Here's how the part is built. I have some questions about the finished solid (model axes, mm). Face numbers are marked on the shaded views. A direction names the side the tool comes from. Coordinates: 2 decimals unless noted, no trailing zeros. Write each loop counter-clockwise with the first axis right and the second up, starting at its lowest first coordinate (ties: lowest second). Pieces come first, ordered by that corner, then holes. Notation, with made-up numbers: (42.25, 3.25) -> (70.25, 3.25) arc R6 ccw to (70.25, 11.25) -> close; hole circle Ø10 at (-21, 64). An arc over 180 degrees is marked (long way). Use CSV: the item, a comma, the result in double quotes. Start each with the question number.
```python
from build123d import *

# Parameters (mm, degrees)
F0_R     = 11.125
F1_DEPTH = 7
F2_DEPTH = 7
F3_DEPTH = 7


with BuildPart() as f1:
    # F0 (on Top) → F1 (new body)
    with BuildSketch(Plane.XY):
        with BuildLine():
            Line((14.352928, 23.6), (0.942339, 49.019534))
            Line((0.942339, 49.019534), (-6.80188, 35.797903))
            Line((-6.80188, 35.797903), (-14.258011, 23.764401))
            Line((-14.258011, 23.764401), (-9.599727, 15.550613))
            ThreePointArc((-9.599727, 15.550613), (-8.984191, 12.491637), (-10.302184, 9.663366))
            ThreePointArc((-10.302184, 9.663366), (-12.214839, 7.093189), (-13.499103, 4.158105))
            ThreePointArc((-13.499103, 4.158105), (-15.307655, 1.607595), (-18.277547, 0.63))
            Line((-18.277547, 0.63), (-27.614663, 0.63))
            Line((-27.614663, 0.63), (-42.923331, -23.693677))
            Line((-42.923331, -23.693677), (-27.600953, -23.789553))
            Line((-27.600953, -23.789553), (-13.45157, -24.23))
            Line((-13.45157, -24.23), (-8.667362, -16.088915))
            ThreePointArc((-8.667362, -16.088915), (-6.325979, -14.026356), (-3.217628, -13.753636))
            ThreePointArc((-3.217628, -13.753636), (-0.035463, -14.124955), (3.148527, -13.769619))
            ThreePointArc((3.148527, -13.769619), (6.261609, -14.060615), (8.593178, -16.14382))
            Line((8.593178, -16.14382), (13.261736, -24.23))
            Line((13.261736, -24.23), (41.980992, -25.325857))
            Line((41.980992, -25.325857), (27.70958, 0.465599))
            Line((27.70958, 0.465599), (18.26709, 0.538301))
            ThreePointArc((18.26709, 0.538301), (15.31017, 1.534719), (13.519812, 4.09027))
            ThreePointArc((13.519812, 4.09027), (12.250302, 7.031766), (10.350576, 9.611514))
            ThreePointArc((10.350576, 9.611514), (9.046046, 12.45302), (9.68437, 15.51382))
            Line((9.68437, 15.51382), (14.352928, 23.6))
        make_face()
        Polygon((-31.423317, -11.732377), (-25.872195, -2.117552), (-13.976091, -2.045608), (-8.500632, -11.280731), (-14.769951, -21.347202), (-25.872195, -21.347202), align=None, mode=Mode.SUBTRACT)
        Polygon((25.872195, -21.347202), (14.769951, -21.347202), (8.759594, -11.080845), (14.019715, -1.721397), (25.872195, -2.117552), (31.423317, -11.732377), align=None, mode=Mode.SUBTRACT)
        Circle(F0_R, mode=Mode.SUBTRACT)
        Polygon((-11.102244, 23.464754), (-5.551122, 33.079579), (5.551122, 33.079579), (11.102244, 23.464754), (5.216496, 13.126454), (-5.519084, 13.002128), align=None, mode=Mode.SUBTRACT)
    extrude(amount=F1_DEPTH)

    # F0 (on Top) → F2 (join)
    with BuildSketch(Plane.XY):
        with BuildLine():
            Line((14.352928, 23.6), (0.942339, 49.019534))
            Line((0.942339, 49.019534), (-6.80188, 35.797903))
            Line((-6.80188, 35.797903), (-14.258011, 23.764401))
            Line((-14.258011, 23.764401), (-9.599727, 15.550613))
            ThreePointArc((-9.599727, 15.550613), (-8.984191, 12.491637), (-10.302184, 9.663366))
            ThreePointArc((-10.302184, 9.663366), (-12.214839, 7.093189), (-13.499103, 4.158105))
            ThreePointArc((-13.499103, 4.158105), (-15.307655, 1.607595), (-18.277547, 0.63))
            Line((-18.277547, 0.63), (-27.614663, 0.63))
            Line((-27.614663, 0.63), (-42.923331, -23.693677))
            Line((-42.923331, -23.693677), (-27.600953, -23.789553))
            Line((-27.600953, -23.789553), (-13.45157, -24.23))
            Line((-13.45157, -24.23), (-8.667362, -16.088915))
            ThreePointArc((-8.667362, -16.088915), (-6.325979, -14.026356), (-3.217628, -13.753636))
            ThreePointArc((-3.217628, -13.753636), (-0.035463, -14.124955), (3.148527, -13.769619))
            ThreePointArc((3.148527, -13.769619), (6.261609, -14.060615), (8.593178, -16.14382))
            Line((8.593178, -16.14382), (13.261736, -24.23))
            Line((13.261736, -24.23), (41.980992, -25.325857))
            Line((41.980992, -25.325857), (27.70958, 0.465599))
            Line((27.70958, 0.465599), (18.26709, 0.538301))
            ThreePointArc((18.26709, 0.538301), (15.31017, 1.534719), (13.519812, 4.09027))
            ThreePointArc((13.519812, 4.09027), (12.250302, 7.031766), (10.350576, 9.611514))
            ThreePointArc((10.350576, 9.611514), (9.046046, 12.45302), (9.68437, 15.51382))
            Line((9.68437, 15.51382), (14.352928, 23.6))
        make_face()
        Polygon((-31.423317, -11.732377), (-25.872195, -2.117552), (-13.976091, -2.045608), (-8.500632, -11.280731), (-14.769951, -21.347202), (-25.872195, -21.347202), align=None, mode=Mode.SUBTRACT)
        Polygon((25.872195, -21.347202), (14.769951, -21.347202), (8.759594, -11.080845), (14.019715, -1.721397), (25.872195, -2.117552), (31.423317, -11.732377), align=None, mode=Mode.SUBTRACT)
        Circle(F0_R, mode=Mode.SUBTRACT)
        Polygon((-11.102244, 23.464754), (-5.551122, 33.079579), (5.551122, 33.079579), (11.102244, 23.464754), (5.216496, 13.126454), (-5.519084, 13.002128), align=None, mode=Mode.SUBTRACT)
    extrude(amount=F2_DEPTH)

    # F0 (on Top) → F3 (join)
    with BuildSketch(Plane.XY):
        with BuildLine():
            Line((14.352928, 23.6), (0.942339, 49.019534))
            Line((0.942339, 49.019534), (-6.80188, 35.797903))
            Line((-6.80188, 35.797903), (-14.258011, 23.764401))
            Line((-14.258011, 23.764401), (-9.599727, 15.550613))
            ThreePointArc((-9.599727, 15.550613), (-8.984191, 12.491637), (-10.302184, 9.663366))
            ThreePointArc((-10.302184, 9.663366), (-12.214839, 7.093189), (-13.499103, 4.158105))
            ThreePointArc((-13.499103, 4.158105), (-15.307655, 1.607595), (-18.277547, 0.63))
            Line((-18.277547, 0.63), (-27.614663, 0.63))
            Line((-27.614663, 0.63), (-42.923331, -23.693677))
            Line((-42.923331, -23.693677), (-27.600953, -23.789553))
            Line((-27.600953, -23.789553), (-13.45157, -24.23))
            Line((-13.45157, -24.23), (-8.667362, -16.088915))
            ThreePointArc((-8.667362, -16.088915), (-6.325979, -14.026356), (-3.217628, -13.753636))
            ThreePointArc((-3.217628, -13.753636), (-0.035463, -14.124955), (3.148527, -13.769619))
            ThreePointArc((3.148527, -13.769619), (6.261609, -14.060615), (8.593178, -16.14382))
            Line((8.593178, -16.14382), (13.261736, -24.23))
            Line((13.261736, -24.23), (41.980992, -25.325857))
            Line((41.980992, -25.325857), (27.70958, 0.465599))
            Line((27.70958, 0.465599), (18.26709, 0.538301))
            ThreePointArc((18.26709, 0.538301), (15.31017, 1.534719), (13.519812, 4.09027))
            ThreePointArc((13.519812, 4.09027), (12.250302, 7.031766), (10.350576, 9.611514))
            ThreePointArc((10.350576, 9.611514), (9.046046, 12.45302), (9.68437, 15.51382))
            Line((9.68437, 15.51382), (14.352928, 23.6))
        make_face()
        Polygon((-31.423317, -11.732377), (-25.872195, -2.117552), (-13.976091, -2.045608), (-8.500632, -11.280731), (-14.769951, -21.347202), (-25.872195, -21.347202), align=None, mode=Mode.SUBTRACT)
        Polygon((25.872195, -21.347202), (14.769951, -21.347202), (8.759594, -11.080845), (14.019715, -1.721397), (25.872195, -2.117552), (31.423317, -11.732377), align=None, mode=Mode.SUBTRACT)
        Circle(F0_R, mode=Mode.SUBTRACT)
        Polygon((-11.102244, 23.464754), (-5.551122, 33.079579), (5.551122, 33.079579), (11.102244, 23.464754), (5.216496, 13.126454), (-5.519084, 13.002128), align=None, mode=Mode.SUBTRACT)
    extrude(amount=F3_DEPTH)


solid = f1.part
```
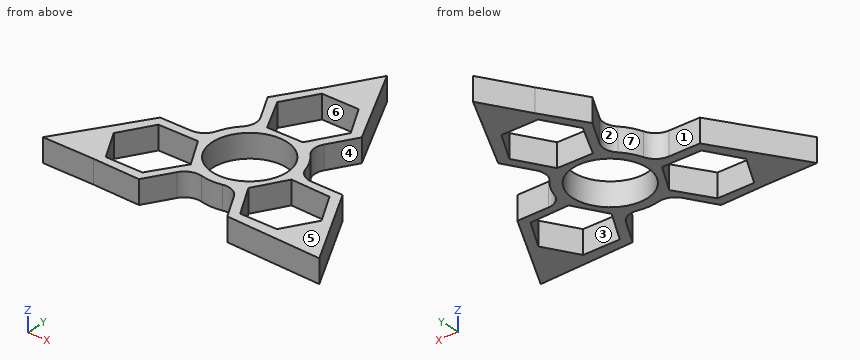
Item 1: I want a section at A-A on x = 0. Please give me the cut outline in (y, z) (3 decimals), then the cut area to 3 significant figures.
Item 2: I want a section at B-B on z = 1.5. Count the separate pieces of the cut face and the enclosed holes in it, then the cut area to 3 significant figures.
Item 3: Thinking about a two-plate mould opening in X: for the marked faces 1, 2 and 3, which applies, +X half, -X half, draft (parallel to the pull), parting line (faces both ways), or undercut?
Item 4: I'm going to push flat-ended pins straight in: pin 1 (1.5 mm diameter, centred on x = -25, z = 6, fed in from +Y); pin 2 (1.5 mm diameter, centred on y = 14.5, z = 2, fed in from -X); pin 3 (3 mm diameter, centred on y = 33.5, z = 6, fed in from -X); pin 4 (1 mm diameter, centred on x = 30.5, y = -11.5, fed in from +Z). Where does each tip first touch, or does it pass through?
Item 5: If I drill on line 1 along X through (y, z) = (-9, 0.75); line 2 along Y through (x, z) = (0, 3.75) (3 decimals); line 3 along X through (y, z) = (-16.5, 0.5), over which ranges is the centre line in solid material (lowest first)?
Item 6: I want a section at C-C on x = -38. Please give me the cut outline in (y, z), then the cut area to 3 significant figures.
Item 7: Which directions (+Z, -Z, +X, -X, +Y, -Y) give clear straight access to the entire face, cutting with the end or side of a thin tool? Please do the marked faces 4, 5, 6 and 7.
Geometry says:
1,outline,"(-14.125, 0) -> (-11.125, 0) -> (-11.125, 7) -> (-14.125, 7) -> close; (11.125, 0) -> (13.066, 0) -> (13.066, 7) -> (11.125, 7) -> close; (33.08, 0) -> (47.411, 0) -> (47.411, 7) -> (33.08, 7) -> close"
1,area,"135 mm2"
2,separate pieces,"1"
2,enclosed holes,"4"
2,area,"1,050 mm2"
3,face 1,"draft"
3,face 2,"-X half"
3,face 3,"undercut"
4,pin 1,"y = 0.63"
4,pin 2,"x = -9.44"
4,pin 3,"x = -9.16"
4,pin 4,"through"
5,line 1,"-33.68 to -29.85, -9.85 to -6.54, 6.54 to 9.93, 29.85 to 32.95"
5,line 2,"-14.125 to -11.125, 11.125 to 13.066, 33.08 to 47.411"
5,line 3,"-38.4 to -28.67, -11.75 to -8.91, 8.8 to 11.93, 28.67 to 37.1"
6,outline,"(-23.72, 0) -> (-15.87, 0) -> (-15.87, 7) -> (-23.72, 7) -> close"
6,area,"55.0 mm2"
7,face 4,"+Z, -Z, +X"
7,face 5,"+Z, +X, -X, +Y, -Y"
7,face 6,"+Z, -Z"
7,face 7,"+Z, -Z, -X"
